from build123d import *

# Parameters (mm, degrees)
SKETCH_1_R          = 1
EXTRUDE_2_DEPTH     = 4
EXTRUDE_3_DEPTH     = 1
CUT_EXTRUDE_2_DEPTH = 1


with BuildPart() as part:
    # 草图1 → 凸台-拉伸2 (new body)
    with BuildSketch(Plane(origin=(0, 0, 0), x_dir=(1, 0, 0), z_dir=(0, 1, 0))):
        Polygon((-24.994291736, 0), (11.005708264, 0), (11.005708264, 1), (16.005708264, 1), (16.005708264, -9), (11.005708264, -9), (11.005708264, -8), (-24.994291736, -8), (-24.994291736, -9), (-29.994291736, -9), (-29.994291736, 1), (-24.994291736, 1), align=None)
        with Locations((-27.994291736, -6.5)):
            Circle(SKETCH_1_R, mode=Mode.SUBTRACT)
        with Locations((-27.994291736, -1.5)):
            Circle(SKETCH_1_R, mode=Mode.SUBTRACT)
        with Locations((14.005708264, -1.5)):
            Circle(SKETCH_1_R, mode=Mode.SUBTRACT)
        with Locations((14.005708264, -6.5)):
            Circle(SKETCH_1_R, mode=Mode.SUBTRACT)
    extrude(amount=EXTRUDE_2_DEPTH)

    # 草图2 → 凸台-拉伸3 (add)
    with BuildSketch(Plane(origin=(0, 4, 0), x_dir=(1, 0, 0), z_dir=(0, 1, 0))):
        with BuildLine():
            Line((-14.894291736, -1.75), (0.905708264, -1.75))
            ThreePointArc((0.905708264, -1.75), (3.155708264, -4), (0.905708264, -6.25))
            Line((0.905708264, -6.25), (-14.894291736, -6.25))
            ThreePointArc((-14.894291736, -6.25), (-17.144291736, -4), (-14.894291736, -1.75))
        make_face()
    extrude(amount=EXTRUDE_3_DEPTH)

    # 草图3 → 切除-拉伸2 (cut)
    with BuildSketch(Plane(origin=(0, 5, 0), x_dir=(1, 0, 0), z_dir=(0, 1, 0))):
        with BuildLine():
            Line((-14.894291736, -2.5), (-14.894291736, -1.75))
            Line((-14.894291736, -1.75), (0.905708264, -1.75))
            Line((0.905708264, -1.75), (0.905708264, -2.5))
            ThreePointArc((0.905708264, -2.5), (2.405708264, -4), (0.905708264, -5.5))
            Line((0.905708264, -5.5), (0.905708264, -6.25))
            Line((0.905708264, -6.25), (-14.894291736, -6.25))
            Line((-14.894291736, -6.25), (-14.894291736, -5.5))
            ThreePointArc((-14.894291736, -5.5), (-16.394291736, -4), (-14.894291736, -2.5))
        make_face()
    extrude(amount=-CUT_EXTRUDE_2_DEPTH, mode=Mode.SUBTRACT)

    # 切除-扫描2: sweep along a path in 草图5
    with BuildLine(Plane(origin=(0, 5, 0), x_dir=(1, 0, 0), z_dir=(0, 1, 0))) as sweep_2_path:
        CenterArc((-14.894291736, -4), 2.25, 0, 360)
    # 草图4 → 切除-扫描2 (sweep, cut)
    with BuildSketch(Plane(origin=(-14.894291736, 0, 0), x_dir=(0, 0, -1), z_dir=(1, 0, 0))):
        with BuildLine():
            Line((-6.25, 5), (-6.25, 4))
            add(Edge.make_bspline(
                [(-6.25, 5), (-5.95, 4.5), (-6.25, 4)],
                knots=[0, 0, 0, 1, 1, 1], degree=2))
        make_face()
    sweep(path=sweep_2_path.line, mode=Mode.SUBTRACT)

    # 切除-扫描3: sweep along a path in 草图9
    with BuildLine(Plane(origin=(0, 5, 0), x_dir=(1, 0, 0), z_dir=(0, 1, 0))) as sweep_3_path:
        CenterArc((0.905708264, -4), 2.25, 0, 360)
    # 草图8 → 切除-扫描3 (sweep, cut)
    with BuildSketch(Plane.ZY.offset(-0.905708264)):
        with BuildLine():
            Line((6.25, 4), (6.25, 5))
            add(Edge.make_bspline(
                [(6.25, 4), (5.95, 4.5), (6.25, 5)],
                knots=[0, 0, 0, 1, 1, 1], degree=2))
        make_face()
    sweep(path=sweep_3_path.line, mode=Mode.SUBTRACT)


solid = part.part
Geometry: final body of the model. Coordinates: model frame, mm. A direction names the side the tool comes from. Give positions to 0.01 mm unless a question says otherwise; leave off trailing zeros. Write each loop counter-clockwise with the first axis right and the second up, starting at its lowest first coordinate (ties: lowest second). Pieces come first, ordered by that corner, then holes.
(1) Ray query, line 1 (X direction, y = 2.9, z = 1.5); line 2 (X direction, y = 1.9, z = 7.25); line 3 (Y direction, x = -7.5, z = 6). Return the intervals inside material, ascending.
(2) Cut plane A-A, the plane y = 2. Return loops of the section in (x, z), then the cut area to 3 significant figures.
(3) Cut plane B-B, the plane z = 7. Return loops of the section in (x, y).
(4) First-contact query: P1, Ø5, axis at x = -21.5, z = 1.5, coming from the +Y side; P2, Ø0.6, axis at y = 4.5, z = 2, coming from the -X side; P3, Ø1.2, axis at x = 14.01, z = 1.5, coming from the -Y side; P4, Ø1.5, axis at x = -22.5, y = 4, coming from the +Z side. Flat tips, straight axial feed; report the tip coordinate or a pass-through.
(5) Cut plane C-C, the plane x = 4. Return loops of the section in (y, z).
(6) Mould query, pull axis Z, two halves, no side actions, for faces 1 (the flat face through (-24.994, 2, 8.5)), 2 (the cylindrical face through (13.007, 1.972, 1.456)), 3 (the flat face through (13, 2, -1)). Classes: released by +Z, released by -Z, zero draft, split by the parting line, or undercut.
(7) Access query for faces 4 (the flat face through (-28, 2, -1)), 5 (the cylindrical face through (2.405, 4.507, 3.967)), 6 (the flat face through (11.006, 2, -0.5)), 7 (the flat face through (-7, 2, 8)), 8 (the flat face through (16.006, 2, 4)). Directions: +Z, -Z, +X, -X, +Y, -Y. A direction counts if a zero-diameter tool reaches every point of the face in a straight line with its end or side. Return the directions, or none.
Values follow:
1. line 1: x = -29.99 to -28.99, -26.99 to 13.01, 15.01 to 16.01
1. line 2: x = -29.99 to -28.66, -27.33 to 13.34, 14.67 to 16.01
1. line 3: y = 0 to 4
2. outline: (-29.99, -1) - (-24.99, -1) - (-24.99, 0) - (11.01, 0) - (11.01, -1) - (16.01, -1) - (16.01, 9) - (11.01, 9) - (11.01, 8) - (-24.99, 8) - (-24.99, 9) - (-29.99, 9) - close; hole circle Ø2 at (-27.99, 1.5); hole circle Ø2 at (-27.99, 6.5); hole circle Ø2 at (14.01, 1.5); hole circle Ø2 at (14.01, 6.5)
2. area: 375 mm2
3. outline: (-29.99, 0) - (-28.86, 0) - (-28.86, 4) - (-29.99, 4) - close; (-27.13, 0) - (13.14, 0) - (13.14, 4) - (-27.13, 4) - close; (14.87, 0) - (16.01, 0) - (16.01, 4) - (14.87, 4) - close
4. P1: stops at y = 4
4. P2: stops at x = -16.13
4. P3: passes through
4. P4: stops at z = 8
5. outline: (0, 0) - (4, 0) - (4, 8) - (0, 8) - close
6. face 1: zero draft
6. face 2: undercut
6. face 3: released by -Z
7. face 4: -Z, +X, -X, +Y, -Y
7. face 5: +Y
7. face 6: -Z, +Y, -Y
7. face 7: +Z, +Y, -Y
7. face 8: +Z, -Z, +X, +Y, -Y
